Verification items for this drawing (mm, ordinates from the low corner). A direction names the side the tool comes from. Round coordinates to 2 decimals unless told otherwise and drop trailing zeros. Write each loop counter-clockwise with the first axis right and the second up, starting at its lowest first coordinate (ties: lowest second). Pieces come first, ordered by that corner, then holes.
Item 1: Cross-section at D-D (z = 10). Enter the section's corners in (x, y).
Item 2: Cross-section at C-C (x = 38). Enter the section's corners in (y, z), then the cut area to 3 significant figures.
Item 3: Depth check by flat-ended pin: P1, Ø7.5, axis at x = 2, z = 5.5, coming from the +Y side; P2, Ø2.5, axis at y = 36, z = 11.5, coming from the +X side; P3, Ø6, axis at y = 14.5, z = 11, coming from the -X side. Enter the tip coordinate at first touch or a pass-through.
Item 4: Scan lines: probe 1 along X at (y, z) = (28.9, 5); probe 2 along Z at (x, y) = (2.5, 28.15); probe 3 along Y at (x, z) = (39, 3.75). Record each from-to range of solid material in increasing order.
Item 5: Cross-section at B-B (x = 51.5). Enter the section's corners in (y, z).
Item 6: Access from +Z, -Z, +X, -X, +Y, -Y to the whole of each face (thin tool, end or side, straight path). Record for the marked faces 1, 2 and 3.
Item 7: Cross-section at A-A (z = 5). Enter the section's corners in (x, y), then the cut area to 3 significant figures.
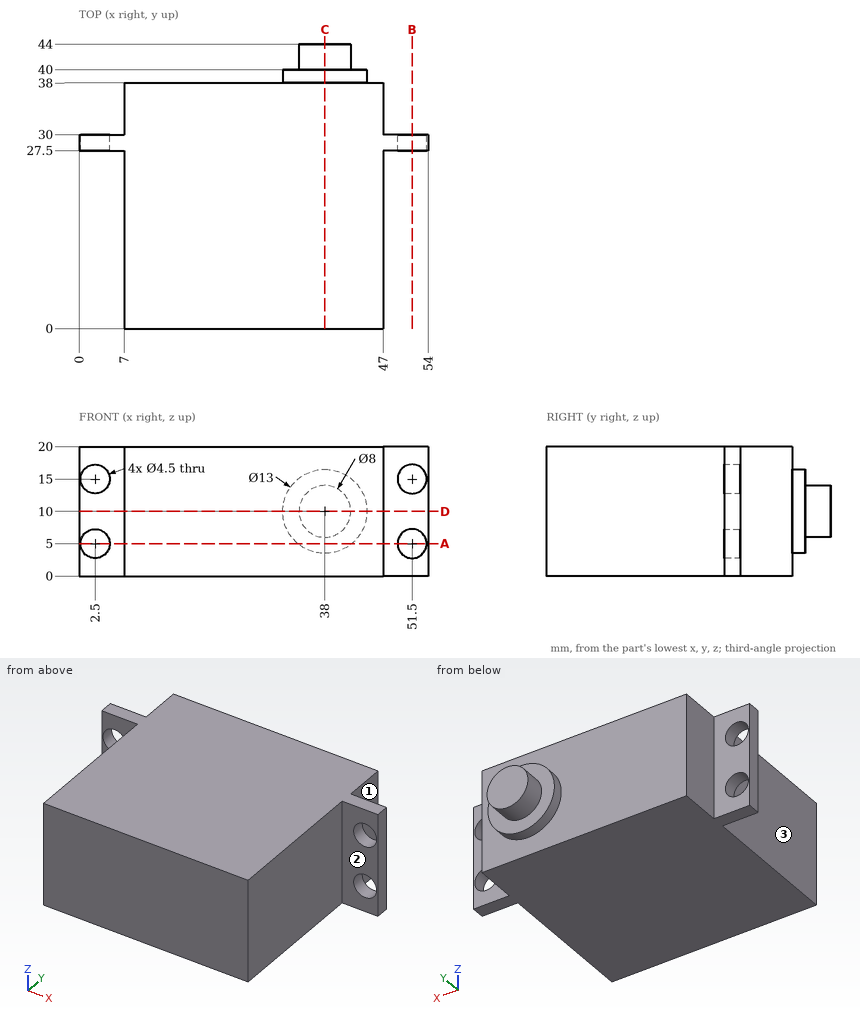
Resolved:
1. outline: (0, 27.5) - (7, 27.5) - (7, 0) - (47, 0) - (47, 27.5) - (54, 27.5) - (54, 30) - (47, 30) - (47, 38) - (44.5, 38) - (44.5, 40) - (42, 40) - (42, 44) - (34, 44) - (34, 40) - (31.5, 40) - (31.5, 38) - (7, 38) - (7, 30) - (0, 30) - close
2. outline: (0, 0) - (38, 0) - (38, 3.5) - (40, 3.5) - (40, 6) - (44, 6) - (44, 14) - (40, 14) - (40, 16.5) - (38, 16.5) - (38, 20) - (0, 20) - close
2. area: 818 mm2
3. P1: stops at y = 30
3. P2: stops at x = 47
3. P3: stops at x = 7
4. probe 1: x = 0 to 0.25, 4.75 to 49.25, 53.75 to 54
4. probe 2: z = 0 to 2.75, 7.25 to 12.75, 17.25 to 20
4. probe 3: y = 0 to 40
5. outline: (27.5, 0) - (30, 0) - (30, 2.75) - (27.5, 2.75) - close; (27.5, 7.25) - (30, 7.25) - (30, 12.75) - (27.5, 12.75) - close; (27.5, 17.25) - (30, 17.25) - (30, 20) - (27.5, 20) - close
6. face 1: +Z, -Z, +X, +Y
6. face 2: +Z, -Z, +X, -Y
6. face 3: +Z, -Z, -X, -Y
7. outline: (0, 27.5) - (0.25, 27.5) - (0.25, 30) - (0, 30) - close; (4.75, 27.5) - (7, 27.5) - (7, 0) - (47, 0) - (47, 27.5) - (49.25, 27.5) - (49.25, 30) - (47, 30) - (47, 38) - (42.15, 38) - (42.15, 40) - (33.85, 40) - (33.85, 38) - (7, 38) - (7, 30) - (4.75, 30) - close; (53.75, 27.5) - (54, 27.5) - (54, 30) - (53.75, 30) - close
7. area: 1,550 mm2
